from build123d import *

# Parameters (mm, degrees)
EXTRUDE_738_DEPTH          = 7.5
HOLE_WIZARD_M8_D           = 6.8
HOLE_WIZARD_M8_DEPTH       = 30
HOLE_WIZARD_M8_TIP         = 2.042926105
HOLE_WIZARD_M12_AT_2_COUNT = 2
HOLE_WIZARD_M12_AT_2_PITCH = 40
HOLE_WIZARD_M12_AT_3_COUNT = 2
HOLE_WIZARD_M12_AT_3_PITCH = 56.568542495
SKETCH_12_R                = 14
CUT_EXTRUDE_1_DEPTH        = 328.504072273
FF10_M3_D                  = 2.5
FF10_M3_CSINK_D            = 3.05
FF10_M3_CSINK_ANGLE        = 90


with BuildPart() as part:
    # Эскиз1 → Extrude 738 (new, symmetric)
    with BuildSketch(Plane(origin=(0, 0, 0), x_dir=(0, 0, -1), z_dir=(1, 0, 0))):
        Polygon((-80, 0), (0, 0), (80, 0), (80, 8), (200, 138.909090909), (200, 258.909090909), (150, 258.909090909), (-80, 8), align=None)
    extrude(amount=EXTRUDE_738_DEPTH, both=True)

    # Крепление к плите M8
    with Locations(Plane(origin=(0, 0, 0), x_dir=(-1, 0, 0), z_dir=(0, -1, 0))):
        with Locations((0, -50), (0, 50)):
            Hole(HOLE_WIZARD_M8_D / 2, depth=HOLE_WIZARD_M8_DEPTH)
            with Locations((0, 0, -(HOLE_WIZARD_M8_DEPTH + HOLE_WIZARD_M8_TIP / 2))):  # 118° drill point
                Cone(0, HOLE_WIZARD_M8_D / 2, HOLE_WIZARD_M8_TIP, mode=Mode.SUBTRACT)

    # Эскиз9 → К профилю M12 (revolve, cut)
    with BuildSketch(Plane(origin=(-7.5, 196.809090909, -180), x_dir=(0, 0, 1), z_dir=(0, 1, 0))):
        Polygon((0, 0), (0, 15), (6.75, 15), (6.75, 6), (10, 6), (10, 0.025), (10.025, 0), align=None)
    hole_wizard_m12 = revolve(axis=Axis((-13.85, 196.809090909, -180), (1, 0, 0)), mode=Mode.SUBTRACT)

    # К профилю M12 at 2: К профилю M12 ×2
    with Locations(*[(0, -i * HOLE_WIZARD_M12_AT_2_PITCH, 0) for i in range(1, HOLE_WIZARD_M12_AT_2_COUNT)]):
        add(hole_wizard_m12, mode=Mode.SUBTRACT)

    # К профилю M12 at 3: К профилю M12 ×2
    with Locations(*[Vector(0, -0.7071067811865478, 0.7071067811865474) * (i * HOLE_WIZARD_M12_AT_3_PITCH) for i in range(1, HOLE_WIZARD_M12_AT_3_COUNT)]):
        add(hole_wizard_m12, mode=Mode.SUBTRACT)

    # Эскиз12 → Вырез-Вытянуть1 (cut, through all)
    with BuildSketch(Plane.ZY.offset(7.5)):
        with Locations((-140, 203.31)):
            Circle(SKETCH_12_R)
    extrude(amount=-CUT_EXTRUDE_1_DEPTH, mode=Mode.SUBTRACT)

    # FF10-M3 (through all)
    with Locations(Plane.ZY.offset(7.5)):
        with Locations((-127.625631329, 215.684368671), (-127.625631329, 190.935631329), (-152.374368671, 190.935631329), (-152.374368671, 215.684368671)):
            CounterSinkHole(FF10_M3_D / 2, FF10_M3_CSINK_D / 2, counter_sink_angle=FF10_M3_CSINK_ANGLE)


solid = part.part
Geometry check sheet. Reference: the model listing, model coordinates, mm. A direction names the side the tool comes from. Give positions to 0.01 mm unless a question says otherwise; leave off trailing zeros. Loops run counter-clockwise (first coordinate to the right, second up) from the corner with the lowest first, then second, coordinate; pieces in that order, holes last.
(1) Depth check by flat-ended pin: pin 1 Ø9 at (x, y) = (-1, 2.5) entering from -Z; pin 2 Ø17 at (y, z) = (203.31, -140) entering from -X; pin 3 Ø4 at (x, z) = (0, -50) entering from -Y; pin 4 Ø4 at (x, z) = (0, 50) entering from +Y. Enter the tip coordinate at first touch or a pass-through.
From the geometry:
pin 1: stops at z = -80
pin 2: passes through
pin 3: stops at y = 30.84
pin 4: stops at y = 42.91
(2) Section check A-A on z = -140. Record the cut outline in (x, y) (3 decimals).
From the geometry:
outline: (-7.5, 73.455) - (7.5, 73.455) - (7.5, 150.059) - (-1.5, 150.059) - (-1.5, 146.809) - (-7.475, 146.809) - (-7.5, 146.784) - close; (-7.5, 166.834) - (-7.475, 166.809) - (-1.5, 166.809) - (-1.5, 163.559) - (7.5, 163.559) - (7.5, 189.31) - (-7.5, 189.31) - close; (-7.5, 217.31) - (7.5, 217.31) - (7.5, 248) - (-7.5, 248) - close
(3) Thickness scan on L1, parallel to Y at x = -5.75, z = -180; L2, parallel to Y at x = -2.75, z = -181; L3, parallel to Z at x = 0, y = 8.25. Record the ranges inside material, lowest first.
From the geometry:
L1: y = 117.09 to 146.81, 166.81 to 186.81, 206.81 to 258.91
L2: y = 118.18 to 146.86, 166.76 to 186.86, 206.76 to 258.91
L3: z = -80.23 to -53.4, -46.6 to 46.6, 53.4 to 79.77
(4) Section check C-C on z = -180. Record the cut outline in (x, y) (3 decimals).
From the geometry:
outline: (-7.5, 117.091) - (7.5, 117.091) - (7.5, 150.059) - (-1.5, 150.059) - (-1.5, 146.809) - (-7.475, 146.809) - (-7.5, 146.784) - close; (-7.5, 166.834) - (-7.475, 166.809) - (-1.5, 166.809) - (-1.5, 163.559) - (7.5, 163.559) - (7.5, 190.059) - (-1.5, 190.059) - (-1.5, 186.809) - (-7.475, 186.809) - (-7.5, 186.784) - close; (-7.5, 206.834) - (-7.475, 206.809) - (-1.5, 206.809) - (-1.5, 203.559) - (7.5, 203.559) - (7.5, 258.909) - (-7.5, 258.909) - close
(5) Section check D-D on y = 87. Record the cut outline in (x, z), then the cut area to 3 significant figures.
From the geometry:
outline: (-7.5, -152.42) - (7.5, -152.42) - (7.5, 7.58) - (-7.5, 7.58) - close
area: 2,400 mm2
(6) Section check B-B on z = -30. Record the cut outline in (x, y).
From the geometry:
outline: (-7.5, 0) - (7.5, 0) - (7.5, 128) - (-7.5, 128) - close
(7) Set-up check for faces 4 (the cylindrical face through (-0.44, 15.21, 46.63)), 5 (the cylindrical face through (-0.11, 212.77, -150.32)), 6 (the flat face through (-1.5, 159, -187)), 7 (the flat face through (0, 4, -80)): record each of +Z, -Z, +X, -X, +Y, -Y from which the full face is reachable in a straight line by a thin tool's end or side.
From the geometry:
face 4: -Y
face 5: +X, -X
face 6: -X
face 7: -Z, +X, -X, -Y
(8) Release check for a two-part mould opening along X. For faces 1 (the cylindrical face through (-4.529, 160.639, -170.763)), 2 (the flat face through (-1.5, 159, -147)), 3 (the cylindrical face through (-0.44, 15.21, -53.37)) record: released by +X, released by -X, zero draft, split by the parting line, or undercut.
From the geometry:
face 1: zero draft
face 2: released by -X
face 3: undercut
